Check sheet for the modelled part. Datum: model origin and axes. Units: mm. A direction names the side the tool comes from. Round coordinates to 2 decimals unless told otherwise and drop trailing zeros. Loops run counter-clockwise (first coordinate to the right, second up) from the corner with the lowest first, then second, coordinate; pieces in that order, holes last. Notation, with made-up numbers: (42.5, 20.5) - (74.5, 20.5) arc R24 ccw to (74.5, 48.5) - close; hole circle Ø7 at (51, -26). An arc over 180 degrees is marked (long way). Return JSON: item names as keys, results as strings.
from build123d import *

# Parameters (mm, degrees)
F1_DEPTH = 25


with BuildPart() as f1:
    # F0 (on Top) → F1 (new body)
    with BuildSketch(Plane.XY):
        Polygon((51.4127239585, 48.7721934915), (-37.7440825105, 48.7721934915), (-44.5784032345, 48.7721934915), (-44.5784032345, -55.2958585322), (-21.5902365744, -21.1242605001), (-21.5902365744, 19.8816582561), (51.4127239585, 30.571033374), align=None)
        Polygon((99.8647660017, 37.6655682921), (51.4127239585, 30.571033374), (51.4127239585, 23.4723131254), (99.8647660017, 30.1393648456), align=None)
        Polygon((51.4127239585, 23.4723131254), (51.4127239585, 30.571033374), (-21.5902365744, 19.8816582561), (25.3180470318, 19.8816582561), align=None)
        Polygon((-21.5902365744, -21.1242605001), (-44.5784032345, -55.2958585322), (51.4127239585, -55.2958585322), (25.3180470318, -21.1242605001), align=None)
        Polygon((51.4127239585, -55.2958585322), (-44.5784032345, -55.2958585322), (82.2778115873, -68.4372480694), align=None)
        Polygon((99.8647660017, 30.1393648456), (51.4127239585, 23.4723131254), (51.4127239585, -55.2958585322), (82.2778115873, -68.4372480694), (99.8647660017, -70.2591297885), align=None)
        Polygon((154.5605957508, 37.6655682921), (99.8647660017, 37.6655682921), (99.8647660017, 30.1393648456), align=None)
        Polygon((99.8647660017, -70.2591297885), (82.2778115873, -68.4372480694), (99.8647660017, -75.9252235293), align=None)
        Polygon((154.5605957508, 37.6655682921), (99.8647660017, 30.1393648456), (99.8647660017, -70.2591297885), (154.5605957508, -75.9252235293), align=None)
        Polygon((154.5605957508, -75.9252235293), (99.8647660017, -70.2591297885), (99.8647660017, -75.9252235293), align=None)
    extrude(amount=F1_DEPTH)


solid = f1.part
Q1. Sectioned sample at A-A (y = 16.5). Enter the section's corners in (x, z), plus the area to 3 significant figures.
Answer key:
{"outline": "(-44.58, 0) - (-21.59, 0) - (-21.59, 25) - (-44.58, 25) - close; (51.41, 0) - (154.56, 0) - (154.56, 25) - (51.41, 25) - close", "area": "3,150 mm²"}
Q2. Sectioned sample at B-B (z = 15). Enter the section's corners in (x, y), plus the area to 3 significant figures.
Answer key:
{"outline": "(-44.58, -55.3) - (82.28, -68.44) - (99.86, -75.93) - (154.56, -75.93) - (154.56, 37.67) - (99.86, 37.67) - (51.41, 30.57) - (51.41, 48.77) - (-44.58, 48.77) - close; hole (-21.59, -21.12) - (25.32, -21.12) - (51.41, -55.3) - (51.41, 23.47) - (25.32, 19.88) - (-21.59, 19.88) - close", "area": "18,200 mm²"}
Q3. Tool access check on faces 1 (the face through (51.413, 40, 12)), 2 (the face through (38.18, 21.65, 12.32)), 3 (the face through (54, -13, 0)), 4 (the face through (128, 37.666, 12)). Record the directions out of +Z, -Z, +X, -X, +Y, -Y that give a thin tool (end or side, any length) a straight path to the whole face; none if there is none.
Answer key:
{"face 1": "+Z, -Z, +Y", "face 2": "+Z, -Z", "face 3": "-Z, +X, -X, +Y, -Y", "face 4": "+Z, -Z, +X, +Y"}
Q4. Sectioned sample at D-D (x = 119). Enter the section's corners in (y, z), plus the area to 3 significant figures.
Answer key:
{"outline": "(-75.93, 0) - (37.67, 0) - (37.67, 25) - (-75.93, 25) - close", "area": "2,840 mm²"}
Q5. Sectioned sample at C-C (x = 32.5). Enter the section's corners in (y, z).
Answer key:
{"outline": "(-63.28, 0) - (-30.53, 0) - (-30.53, 25) - (-63.28, 25) - close; (20.87, 0) - (48.77, 0) - (48.77, 25) - (20.87, 25) - close"}
Q6. Draft check along X on faces 5 (the face through (90.95, -72.13, 12.32)), 6 (the face through (127, -75.925, 12)), 7 (the face through (51.413, -15, 12)), 8 (the face through (2, 19.882, 12)). Enter one of: released by +X, released by -X, zero draft, split by the parting line, or undercut.
Answer key:
{"face 5": "released by -X", "face 6": "zero draft", "face 7": "undercut", "face 8": "undercut"}
Q7. Scan lines: probe 1 along X at (y, z) = (-9, 1); probe 2 along X at (y, z) = (44.5, 5.75); probe 3 along Y at (x, z) = (-15, 22.5). Record each from-to range of solid material in increasing order. Write a range as [from, to].
Answer key:
{"probe 1": "x = [-44.58, -21.59], [51.41, 154.56]", "probe 2": "x = [-44.58, 51.41]", "probe 3": "y = [-58.36, -21.12], [19.88, 48.77]"}
